Part model, mm, in its own coordinate system. A direction names the side the tool comes from. Coordinates: 2 decimals unless noted, no trailing zeros. Order: outer loops, then holes, each group sorted by start corner. A loop starts at its lowest first (then second) coordinate and runs counter-clockwise, first axis right, second up. Notation, with made-up numbers: M 24.25,-33 L 71.25,-33 A15 ccw 71.25,-13 Z; hole C 34.25,75.5 d1. An arc over 180 degrees is marked long. Answer in a Markdown table with one row per item. Add a question column.
Autodesk Inventor part; units mm, degrees
ref_plane "YZ Plane" through (0, 0, 0) normal (1, 0, 0) x (0, 1, 0)
ref_plane "XZ Plane" through (0, 0, 0) normal (0, 1, 0) x (-1, 0, 0)
ref_plane "XY Plane" through (0, 0, 0) normal (0, 0, 1) x (1, 0, 0)
sketch "Sketch1" plane through (0, 0, 0) normal (0, 0, 1) x (1, 0, 0)
  line L0 (0, 0) -> (230, 0)
  line L1 (230, 0) -> (230, 20)
  line L2 (230, 20) -> (0, 20)
  line L3 (0, 20) -> (0, 0)
  dimension "d0" = 230
  dimension "d1" = 20
extrude "Extrusion1" add sketch "Sketch1" along normal blind 3
sketch "Sketch2" plane through (0, 0, 3) normal (0, 0, -1) x (-1, 0, 0)
  line L0 (0, 0) -> (-230, 0)
  line L1 (-12.5251, -24.7625) -> (-37.9251, -24.7625)
  line L2 (-230, 20) -> (0, 20)
  point P0 (-10.225, 30)
  dimension "d62" = 10
  dimension "d73" = 10.225
sketch "Sketch5" plane through (0, 0, 0) normal (-1, 0, 0) x (0, 0, 1)
  line L0 (0, 20) -> (3, 20)
  line L1 (3, 20) -> (-7, 20)
  line L2 (-7, 20) -> (-7, 40)
  line L3 (-7, 40) -> (3, 40)
  line L4 (3, 40) -> (3, 20)
  point P0 (0, 0)
  point P1 (3, 30)
  point P2 (1.5, 20)
  point P3 (0, 20)
  dimension "d31" = 10
  dimension "d32" = 20
extrude "Extrusion3" add sketch "Sketch5" against normal up to surface (230 mm away)
hole "Hole3" at (10.225, 30, 3) direction (0, 0, -1) diameter 4.1 depth 6
sketch "Sketch6" plane through (0, 0, 3) normal (0, 0, 1) x (1, 0, 0)
  line L0 (0, 0) -> (0, 40)
  line L1 (230, 0) -> (230, 40)
  line L2 (0, 40) -> (230, 40)
  point P0 (27.6875, 30)
  dimension "d35" = 27.6875
  dimension "d51" = 10
hole "Hole2" at (27.6875, 30, 3) direction (0, 0, -1) diameter 6 end through all
pattern_linear "Rectangular Pattern2" count 6 spacing 34.925 along (1, 0, 0) of "Hole2"
pattern_linear "Rectangular Pattern3" count 7 spacing 34.925 along (1, 0, 0) of "Hole3"
sketch "Sketch7" plane through (0, 0, 0) normal (-1, 0, 0) x (0, 0, 1)
  line L0 (0, 0) -> (3, 0)
  line L1 (0, 0) -> (3.6796, 0)
  line L2 (3.6796, 0) -> (3.6796, 5)
  line L3 (3.6796, 5) -> (0, 5)
  line L4 (0, 5) -> (0, 0)
  dimension "d66" = 5
properties part number "IR_Mount_Plate_3DPrint"
(1) Drop flat-ended pins along their axis: P1, Ø1, axis at x = 195, y = 5.5, coming from the -Z side; P2, Ø5, axis at x = 202.31, y = 30, coming from the +Z side; P3, Ø4.5, axis at x = 184.85, y = 30, coming from the +Z side; P4, Ø3, axis at x = 60.5, z = -3.5, coming from the -Y side. Give the stop position or say it passes through.
(2) Pull direction Y, two halves, no side cores. Call faces 1 (the flat face through (113, 10, 0)), 2 (the flat face through (113, 20, -3)), 3 (the flat face through (113, 40, -2)), 4 (the cylindrical face through (135.39, 30.65, -2.07)): pulls with the +Y half, pulls with the -Y half, needs draft (parallel to the pull), parting line crosses it, or undercut.
(3) Slice it at B-B (x = 15.5). List the corners of the cut face in (y, z).
(4) Slice it at A-A (z = -4.5). List the corners of the cut face in (x, y).
(5) 3-axis set-ups, long thin cutter, end or side, ignore diameter. For faces 5 (the cylindrical face through (221.776, 30.444, -0.042)), 6 (the cylindrical face through (164.413, 30.391, -2.07)): which of +Z, -Z, +X, -X, +Y, -Y reach the whole face in a straight line?
(6) Wall check: line 1 (Z direction, x = 24, y = 19.5); line 2 (Y direction, x = 105, z = -0.5); line 3 (Y direction, x = 186, z = -1.25). Give the ranges that are in metal, low to high.
(7) Slice it at D-D (x = 115). List the corners of the cut face in (y, z).
(8) Slice it at C-C (y = 30). State how many separate pieces and enclosed holes the cut face has, and give its area (3 significant figures).
Computed:
| question | item | result |
|---|---|---|
| 1 | P1 | stops at z = 0 |
| 1 | P2 | passes through |
| 1 | P3 | stops at z = 3 |
| 1 | P4 | stops at y = 20 |
| 2 | face 1 | needs draft |
| 2 | face 2 | pulls with the -Y half |
| 2 | face 3 | pulls with the +Y half |
| 2 | face 4 | undercut |
| 3 | outline | M 0,0 L 20,0 L 20,-7 L 40,-7 L 40,3 L 0,3 Z |
| 4 | outline | M 0,20 L 230,20 L 230,40 L 0,40 Z; hole C 27.69,30 d6; hole C 62.61,30 d6; hole C 97.54,30 d6; hole C 132.46,30 d6; hole C 167.39,30 d6; hole C 202.31,30 d6 |
| 5 | face 5 | +Z |
| 5 | face 6 | +Z, -Z |
| 6 | line 1 | z = 0 to 3 |
| 6 | line 2 | y = 20 to 40 |
| 6 | line 3 | y = 20 to 28.3, 31.7 to 40 |
| 7 | outline | M 0,0 L 20,0 L 20,-7 L 40,-7 L 40,3 L 32.05,3 L 32.05,-3 L 27.95,-3 L 27.95,3 L 0,3 Z |
| 8 | separate pieces | 7 |
| 8 | enclosed holes | 0 |
| 8 | area | 1,770 mm^2 |
